from build123d import *

# Parameters (mm, degrees)
SKETCH1_W           = 10
SKETCH1_H           = 20
BOSS_EXTRUDE1_DEPTH = 4
SKETCH2_R           = 1.6
CUT_EXTRUDE1_DEPTH  = 12.874342087
SKETCH3_R           = 1.25
CUT_EXTRUDE2_DEPTH  = 15.696938457
SKETCH4_W           = 2.75
SKETCH4_H           = 10
CUT_EXTRUDE3_DEPTH  = 12.874342087
SKETCH5_W           = 7.25
SKETCH5_H           = 3.5
CUT_EXTRUDE4_DEPTH  = 12.874342087
CHAMFER1_SIZE       = 3.5
FILLET1_R           = 2


with BuildPart() as part:
    # Sketch1 → Boss-Extrude1 (new body)
    with BuildSketch(Plane(origin=(0, 0, 0), x_dir=(0, 1, 0), z_dir=(0, 0, 1))):
        Rectangle(SKETCH1_W, SKETCH1_H)
    extrude(amount=BOSS_EXTRUDE1_DEPTH)

    # Sketch2 → Cut-Extrude1 (cut, through all)
    with BuildSketch(Plane.XY.offset(4)):
        with Locations((-5, 0)):
            Circle(SKETCH2_R)
    extrude(amount=-CUT_EXTRUDE1_DEPTH, mode=Mode.SUBTRACT)

    # Sketch3 → Cut-Extrude2 (cut, through all)
    with BuildSketch(Plane.XZ.offset(5)):
        with Locations((5, 2)):
            Circle(SKETCH3_R)
    extrude(amount=-CUT_EXTRUDE2_DEPTH, mode=Mode.SUBTRACT)

    # Sketch4 → Cut-Extrude3 (cut, through all)
    with BuildSketch(Plane.XY.offset(4)):
        with Locations((8.625, 0)):
            Rectangle(SKETCH4_W, SKETCH4_H)
    extrude(amount=-CUT_EXTRUDE3_DEPTH, mode=Mode.SUBTRACT)

    # Sketch5 → Cut-Extrude4 (cut, through all)
    with BuildSketch(Plane.XY.offset(4)):
        with Locations((3.625, 3.25)):
            Rectangle(SKETCH5_W, SKETCH5_H)
        with Locations((3.625, -3.25)):
            Rectangle(SKETCH5_W, SKETCH5_H)
    extrude(amount=-CUT_EXTRUDE4_DEPTH, mode=Mode.SUBTRACT)

    # Chamfer1
    chamfer1_edges = [part.edges().sort_by_distance(p)[0] for p in [
        (0, 1.5, 2),
        (0, -1.5, 2),
    ]]
    chamfer(chamfer1_edges, length=CHAMFER1_SIZE - 0.0001)  # a hair under: the kernel refuses the full size

    # Fillet1
    fillet1_edges = [part.edges().sort_by_distance(p)[0] for p in [
        (7.25, 0, 4),
    ]]
    fillet(fillet1_edges, radius=FILLET1_R)


solid = part.part
Geometry check sheet. Reference: the model listing, model coordinates, mm. A direction names the side the tool comes from. Coordinates: 2 decimals unless noted, no trailing zeros. Loops run counter-clockwise (first coordinate to the right, second up) from the corner with the lowest first, then second, coordinate; pieces in that order, holes last. Notation, with made-up numbers: (44, -6.5) - (48, -6.5) arc R24 ccw to (48, 25.5) - close; hole circle Ø1 at (71.25, 55). An arc over 180 degrees is marked (long way). Use one line per item in the form item = value. Start each with the question number.
Item 1: Section check B-B, the plane x = -5. Enter the section's corners in (y, z).
Item 2: Mould release check, pull along X, two halves, no side actions. Record for faces 4 (the face through (-6.6, 0.07, 2.03)), 5 (the face through (6.68, 0.02, 3.4)), 6 (the face through (4.84, -0.02, 3.24)), 7 (the face through (-10, 0, 2)): +X half, -X half, draft (parallel to the pull), parting line (faces both ways), or undercut.
Item 3: Tool access check on faces 1 (the face through (6, 1.5, 1)), 2 (the face through (6, -1.5, 1)), 3 (the face through (-5, -5, 2)). Record the directions out of +Z, -Z, +X, -X, +Y, -Y that give a thin tool (end or side, any length) a straight path to the whole face; none if there is none.
Item 4: Gauge pin test, flat ends, axial feed: pin 1 (1.1 mm diameter, centred on x = 5, z = 3, fed in from +Y); pin 2 (1.5 mm diameter, centred on x = 5.5, y = 0, fed in from +Z). Record the tip position at first contact, or that the pin passes through.
Item 5: Section check C-C, the plane z = 1.45. Give the number of separate pieces and of enclosed holes in the cut face, and give its area (3 significant figures).
Item 6: Thickness scan on probe 1 along Y at (x, z) = (-5, 2.95); probe 2 along X at (y, z) = (1, 2.45); probe 3 along Y at (x, z) = (4.25, 3.5). Record the ranges inside material, lowest first.
Item 7: Section check A-A, the plane y = 0. Enter the section's corners in (x, z).
Computed:
q1.outline = (-5, 0) - (-1.6, 0) - (-1.6, 4) - (-5, 4) - close; (1.6, 0) - (5, 0) - (5, 4) - (1.6, 4) - close
q2.face_4 = undercut
q2.face_5 = +X half
q2.face_6 = undercut
q2.face_7 = -X half
q3.face_1 = +Z, -Z, +X, +Y
q3.face_2 = +Z, -Z, +X, -Y
q3.face_3 = +Z, -Z, +X, -X, -Y
q4.pin_1 = 1.5
q4.pin_2 = 4
q5.separate_pieces = 2
q5.enclosed_holes = 1
q5.area = 119 mm2
q6.probe_1 = -5 to -1.6, 1.6 to 5
q6.probe_2 = -10 to -6.25, -3.75 to 3.83, 6.17 to 7.2
q6.probe_3 = -1.5 to 1.5
q7.outline = (-10, 0) - (-6.6, 0) - (-6.6, 4) - (-10, 4) - close; (-3.4, 0) - (7.25, 0) - (7.25, 2) arc R2 ccw to (5.25, 4) - (-3.4, 4) - close; hole circle Ø2.5 at (5, 2)
